from build123d import *

# Parameters (mm, degrees)
F0_W     = 19.05
F0_H     = 19.05
F0_W_2   = 15.875
F0_H_2   = 15.875
F1_DEPTH = 107.95
F2_R     = 1.5875
F3_R     = 1.5875
F4_R     = 3.2385
F4_R_2   = 2.5796875
F5_DEPTH = 19.05
F6_DEPTH = 47.625
F7_DEPTH = 3.175


# Not quite as in the source:
# - a length typed as a fraction of an inch, garbled in the dataset ("3 / 203.2 mm" for 3/8 in), is restored


with BuildPart() as f1:
    # F0 (on Front) → F1 (new body, symmetric)
    with BuildSketch(Plane.XZ):
        Rectangle(F0_W, F0_H)
        with Locations((-0.0127, 0)):
            Rectangle(F0_W_2, F0_H_2, mode=Mode.SUBTRACT)
    extrude(amount=F1_DEPTH, both=True)

    # F2
    f2_edges = [f1.edges().sort_by_distance(p)[0] for p in [
        (-9.525, 0, 9.525),
        (-9.525, 0, -9.525),
        (9.525, 0, -9.525),
        (9.525, 0, 9.525),
    ]]
    fillet(f2_edges, radius=F2_R)

    # F3
    f3_edges = [f1.edges().sort_by_distance(p)[0] for p in [
        (-7.9502, 0, 7.9375),
        (-7.9502, 0, -7.9375),
        (7.9248, 0, 7.9375),
        (7.9248, 0, -7.9375),
    ]]
    fillet(f3_edges, radius=F3_R)

    # F4 (on face) → F5 (cut)
    with BuildSketch(Plane(origin=(-9.525, 0, 0), x_dir=(0, -1, 0), z_dir=(-1, 0, 0))):
        with Locations((-100.0125, 0)):
            Circle(F4_R)
        with Locations((19.05, 0)):
            Circle(F4_R_2)
        with Locations((50.8, 0)):
            Circle(F4_R_2)
    extrude(amount=-F5_DEPTH, mode=Mode.SUBTRACT)

    # F6 (cut): a face of the model
    f6_faces = [f1.faces().sort_by_distance(p)[0] for p in [
        (-8.2196076836, -107.95, 0),
    ]]
    extrude(f6_faces, amount=-F6_DEPTH, mode=Mode.SUBTRACT)

    # F7 (cut): a face of the model
    f7_faces = [f1.faces().sort_by_distance(p)[0] for p in [
        (-8.2196076836, 107.95, 0),
    ]]
    extrude(f7_faces, amount=-F7_DEPTH, mode=Mode.SUBTRACT)


solid = f1.part
Here's how the part is built. I have some questions about the finished solid (model axes, mm). A direction names the side the tool comes from. Give positions to 0.01 mm unless a question says otherwise; leave off trailing zeros. Order: outer loops, then holes, each group sorted by start corner. A loop starts at its lowest first (then second) coordinate and runs counter-clockwise, first axis right, second up. Notation, with made-up numbers: (44.25, 58) -> (80.25, 58) arc R8 ccw to (80.25, 65) -> close; hole circle Ø7 at (45.25, -13.5). An arc over 180 degrees is marked (long way). Use a Markdown table: item, result. Add a question column.
Item 1: I need wall thicknesses on line 1 (X direction, y = 81.5, z = 6) (3 decimals); line 2 (Z direction, x = 3.5, y = 60) (1 decimal); line 3 (X direction, y = 40, z = -6.5) (3 decimals). Which ranges of each line are inside material? Lowest first, please.
Item 2: If we mould it in two halves opening along X, with no side actions, what happens to faces 3 (the face through (9.525, 21, 0)), 4 (the face through (8.71, 97.02, -1.24)), 5 (the face through (7.925, 21, 0))? For each: pulls with the +X half, pulls with the -X half, needs draft (parallel to the pull), parting line crosses it, or undercut.
Item 3: For faces 1 (the face through (0, 21, 9.525)), 2 (the face through (0, 21, 7.938)), which set-ups out of +Z, -Z, +X, -X, +Y, -Y let a thin tool reach every point of the face, with its end or its side?
Item 4: Imagine slicing it at A-A on x = -4.5. Please give me the cut outline in (y, z) (1 decimal), plus the area to 3 significant figures.
Item 5: Imagine slicing it at B-B on z = 5. Please give me the cut outline in (x, y) (3 decimals), plus the area to 3 significant figures.
Data:
| question | item | result |
|---|---|---|
| 1 | line 1 | x = -9.525 to -7.95, 7.925 to 9.525 |
| 1 | line 2 | z = -9.5 to -7.9, 7.9 to 9.5 |
| 1 | line 3 | x = -9.525 to -7.943, 7.918 to 9.525 |
| 2 | face 3 | pulls with the +X half |
| 2 | face 4 | needs draft |
| 2 | face 5 | undercut |
| 3 | face 1 | +Z, +X, -X, +Y, -Y |
| 3 | face 2 | +Y, -Y |
| 4 | outline | (-60.3, -9.5) -> (104.8, -9.5) -> (104.8, -7.9) -> (-60.3, -7.9) -> close; (-60.3, 7.9) -> (104.8, 7.9) -> (104.8, 9.5) -> (-60.3, 9.5) -> close |
| 4 | area | 524 mm² |
| 5 | outline | (-9.525, -60.325) -> (-7.95, -60.325) -> (-7.95, 104.775) -> (-9.525, 104.775) -> close; (7.925, -60.325) -> (9.525, -60.325) -> (9.525, 104.775) -> (7.925, 104.775) -> close |
| 5 | area | 524 mm² |
